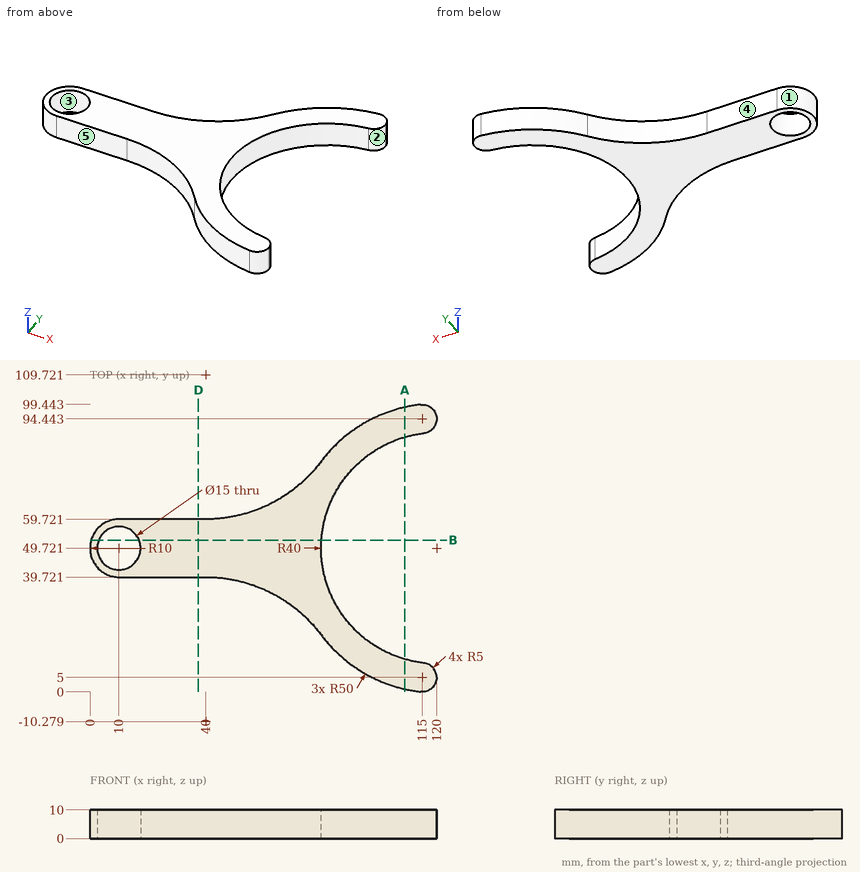
Geometry: see drawing. Coordinates: mm, zero at the bounding-box minimum. A direction names the side the tool comes from. Coordinates: 2 decimals unless noted, no trailing zeros. Order: outer loops, then holes, each group sorted by start corner. A loop starts at its lowest first (then second) coordinate and runs counter-clockwise, first axis right, second up. Notation, with made-up numbers: (5, -10) - (47, -10) arc R11 cw to (47, 2) - close; hole circle Ø2 at (50.25, 4.5). An arc over 180 degrees is marked (long way). Write each question's results on one line, items separated by ' | '.
(1) Set-up query: the marked faces 1 and 2. Return all of +Z, -Z, +X, -X, +Y, -Y with unobstructed straight access to the full face (end or side cutting, diameter ignored); none if empty.
Values found:
face 1: +Z, -Z, -X | face 2: +Z, -Z, +X
(2) Section query D-D, the plane x = 37.5. Return the cut outline in (y, z).
Values found:
outline: (39.72, 0) - (59.72, 0) - (59.72, 10) - (39.72, 10) - close
(3) First-contact query: pin 1 Ø6 at (y, z) = (60, 8.5) entering from -X; pin 2 Ø13.5 at (x, y) = (10, 49.72) entering from -Z; pin 3 Ø5 at (y, z) = (70, 7.5) entering from +X; pin 4 Ø3 at (x, z) = (22.5, 4.5) entering from -Y. Flat tips, straight axial feed; report the tip coordinate or a pass-through.
Values found:
pin 1: stops at x = 3.14 | pin 2: passes through | pin 3: stops at x = 87.12 | pin 4: stops at y = 39.72
(4) Mould query, pull axis Y, two halves, no side actions, for the marked faces 3, 4 and 5. Classes: +Y half, -Y half, draft (parallel to the pull), parting line (faces both ways), or undercut.
Values found:
face 3: undercut | face 4: +Y half | face 5: -Y half
(5) Line query: line 1 (Y direction, x = 10, z = 3.5); line 2 (Y direction, x = 13.5, z = 7) (1 decimal); line 3 (X direction, y = 52, z = 3.5) (1 decimal). Output: solid intervals per line, ascending. Write a range as [from, to].
Values found:
line 1: y = [39.72, 42.22], [57.22, 59.72] | line 2: y = [39.7, 43.1], [56.4, 59.7] | line 3: x = [0.3, 2.9], [17.1, 80.1]
(6) Section query B-B, the plane y = 52.5. Return the cut outline in (x, z).
Values found:
outline: (0.39, 0) - (3.03, 0) - (3.03, 10) - (0.39, 10) - close; (16.97, 0) - (80.1, 0) - (80.1, 10) - (16.97, 10) - close
(7) Section query A-A, the plane x = 109. Return the cut outline in (y, z).
Values found:
outline: (0.95, 0) - (11.26, 0) - (11.26, 10) - (0.95, 10) - close; (88.18, 0) - (98.5, 0) - (98.5, 10) - (88.18, 10) - close
